Can you work these out from the model? Positions are in its coordinate system, mm. Give positions to 0.01 mm unless a question says otherwise; leave off trailing zeros. Loops run counter-clockwise (first coordinate to the right, second up) from the corner with the lowest first, then second, coordinate; pieces in that order, holes last. Notation, with made-up numbers: (62.5, -28.75) -> (73.5, -28.75) arc R22 cw to (73.5, -3.75) -> close; hole circle Ø10 at (60, 74). An arc over 180 degrees is marked (long way). Use CSV: the item, a comma, the result in double quotes.
from build123d import *

# Parameters (mm, degrees)
SKETCH1_R           = 27.5
SKETCH1_R_2         = 8
SKETCH1_R_3         = 1.8
SKETCH1_R_4         = 1.5
BOSS_EXTRUDE1_DEPTH = 6
MOVE_FACE1_BY       = 0.08
MOVE_FACE1_2_BY     = 0.08
MOVE_FACE1_3_BY     = 0.08
MOVE_FACE1_4_BY     = 0.08
MOVE_FACE1_5_BY     = 0.08
MOVE_FACE1_6_BY     = 0.08
MOVE_FACE1_7_BY     = 0.08
MOVE_FACE1_8_BY     = 0.08
MOVE_FACE1_9_BY     = 0.08
MOVE_FACE1_10_BY    = 0.08
MOVE_FACE1_11_BY    = 0.08
MOVE_FACE1_12_BY    = 0.08
MOVE_FACE1_13_BY    = 0.08


with BuildPart() as part:
    # Sketch1 → Boss-Extrude1 (new body)
    with BuildSketch(Plane.XY):
        Circle(SKETCH1_R)
        Circle(SKETCH1_R_2, mode=Mode.SUBTRACT)
        with Locations((0, 23)):
            Circle(SKETCH1_R_3, mode=Mode.SUBTRACT)
        with Locations((0, -23)):
            Circle(SKETCH1_R_3, mode=Mode.SUBTRACT)
        with Locations((-16.263455967, -16.263455967)):
            Circle(SKETCH1_R_4, mode=Mode.SUBTRACT)
        with Locations((-23, 0)):
            Circle(SKETCH1_R_3, mode=Mode.SUBTRACT)
        with Locations((-16.263455967, 16.263455967)):
            Circle(SKETCH1_R_4, mode=Mode.SUBTRACT)
        with Locations((0, 11)):
            Circle(SKETCH1_R_3, mode=Mode.SUBTRACT)
        with Locations((9.526279442, 5.5)):
            Circle(SKETCH1_R_3, mode=Mode.SUBTRACT)
        with Locations((9.526279442, -5.5)):
            Circle(SKETCH1_R_3, mode=Mode.SUBTRACT)
        with Locations((0, -11)):
            Circle(SKETCH1_R_3, mode=Mode.SUBTRACT)
        with Locations((-9.526279442, -5.5)):
            Circle(SKETCH1_R_3, mode=Mode.SUBTRACT)
        with Locations((-9.526279442, 5.5)):
            Circle(SKETCH1_R_3, mode=Mode.SUBTRACT)
    extrude(amount=BOSS_EXTRUDE1_DEPTH)

    # Move Face1: a curved face moved outward by 0.08
    add(Solid.thicken(part.faces().sort_by_distance((-17.763455967, -16.263455967, 3))[0], MOVE_FACE1_BY))

    # Move Face1 2: a curved face moved outward by 0.08
    add(Solid.thicken(part.faces().sort_by_distance((-24.8, 0, 3))[0], MOVE_FACE1_2_BY))

    # Move Face1 3: a curved face moved outward by 0.08
    add(Solid.thicken(part.faces().sort_by_distance((-17.763455967, 16.263455967, 3))[0], MOVE_FACE1_3_BY))

    # Move Face1 4: a curved face moved outward by 0.08
    add(Solid.thicken(part.faces().sort_by_distance((-1.8, 23, 3))[0], MOVE_FACE1_4_BY))

    # Move Face1 5: a curved face moved outward by 0.08
    add(Solid.thicken(part.faces().sort_by_distance((-27.5, 0, 3))[0], MOVE_FACE1_5_BY))

    # Move Face1 6: a curved face moved outward by 0.08
    add(Solid.thicken(part.faces().sort_by_distance((-8, 0, 3))[0], MOVE_FACE1_6_BY))

    # Move Face1 7: a curved face moved outward by 0.08
    add(Solid.thicken(part.faces().sort_by_distance((-1.8, 11, 3))[0], MOVE_FACE1_7_BY))

    # Move Face1 8: a curved face moved outward by 0.08
    add(Solid.thicken(part.faces().sort_by_distance((-1.8, -23, 3))[0], MOVE_FACE1_8_BY))

    # Move Face1 9: a curved face moved outward by 0.08
    add(Solid.thicken(part.faces().sort_by_distance((7.726279442, 5.5, 3))[0], MOVE_FACE1_9_BY))

    # Move Face1 10: a curved face moved outward by 0.08
    add(Solid.thicken(part.faces().sort_by_distance((7.726279442, -5.5, 3))[0], MOVE_FACE1_10_BY))

    # Move Face1 11: a curved face moved outward by 0.08
    add(Solid.thicken(part.faces().sort_by_distance((-1.8, -11, 3))[0], MOVE_FACE1_11_BY))

    # Move Face1 12: a curved face moved outward by 0.08
    add(Solid.thicken(part.faces().sort_by_distance((-11.326279442, -5.5, 3))[0], MOVE_FACE1_12_BY))

    # Move Face1 13: a curved face moved outward by 0.08
    add(Solid.thicken(part.faces().sort_by_distance((-11.326279442, 5.5, 3))[0], MOVE_FACE1_13_BY))


solid = part.part
(1) If we section it at A-A, the plane x = 3: Write out the boundary of the cut face in (y, z).
Answer sheet:
outline,"(-27.42, 0) -> (-7.33, 0) -> (-7.33, 6) -> (-27.42, 6) -> close; (7.33, 0) -> (27.42, 0) -> (27.42, 6) -> (7.33, 6) -> close"
(2) If I drill on L1, parallel to Y at x = 0, z = 1.65; L2, parallel to X at y = 1, z = 5.1; L3, parallel to Y at x = -17.5, z = 5.65, over which ranges is the centre line in solid material (lowest first)? Write a range as from..to.
Answer sheet:
L1,"y = -27.58..-24.72, -21.28..-12.72, -9.28..-7.92, 7.92..9.28, 12.72..21.28, 24.72..27.58"
L2,"x = -27.56..-24.4, -21.6..-7.86, 7.86..27.56"
L3,"y = -21.32..-16.96, -15.57..15.57, 16.96..21.32"
(3) We'd pull the mould along Y, two halves only. Please class faces 1 (the face through (9.302, 7.205, 2.958)), 2 (the face through (6, -6, 6)), 3 (the face through (26.3, 8.3, 3)): released by +Y, released by -Y, zero draft, split by the parting line, or undercut.
Answer sheet:
face 1,"undercut"
face 2,"zero draft"
face 3,"split by the parting line"
(4) If we section it at C-C, the plane z = 1.4: Give the number of separate pieces and of enclosed holes in the cut face, then the cut area to 3 significant figures.
Answer sheet:
separate pieces,"1"
enclosed holes,"12"
area,"2,100 mm2"
(5) If we section it at D-D, the plane x = 13: Write out the boundary of the cut face in (y, z).
Answer sheet:
outline,"(-24.32, 0) -> (24.32, 0) -> (24.32, 6) -> (-24.32, 6) -> close"
(6) Will these pins go through, and if not, where does the flat tip stop? pin 1 Ø2 at (y, z) = (-19, 5) entering from -X; pin 2 Ø3 at (x, y) = (-23, 0) entering from -Z; pin 3 Ø3 at (y, z) = (19.5, 2) entering from +X; pin 4 Ø2 at (x, z) = (-12, 2.5) entering from -Y.
Answer sheet:
pin 1,"stops at x = -20.9"
pin 2,"passes through"
pin 3,"stops at x = 20.9"
pin 4,"stops at y = -25.29"
